Could you check a few things on this model? Use its own coordinates, in mm. A direction names the side the tool comes from. Coordinates: 2 decimals unless noted, no trailing zeros. Order: outer loops, then holes, each group sorted by start corner. A loop starts at its lowest first (then second) coordinate and runs counter-clockwise, first axis right, second up. Notation, with made-up numbers: M 64,43.5 L 94,43.5 A29 cw 94,74.5 Z; hole C -34,36.5 d10. An arc over 180 degrees is marked long. Put each result on its own line as item: value. Start each with the question number.
Autodesk Fusion 360 part; units mm, degrees
sketch "草图1" plane through (0, 0, 0) normal (0, 1, 0) x (1, 0, 0)
  circle A0 centre (0, 0) radius 12
  line L0 (-8.5, -18) -> (8.5, -18)
  line L1 (8.5, -18) -> (15, -4.0607)
  line L2 (-8.5, -18) -> (-15, -4.0607)
  line L3 (0, -38) -> (0, 21) construction
  line L4 (-34, 0) -> (39, 0) construction
  line L5 (-15, 0) -> (-15, -4.0607)
  line L6 (15, 0) -> (15, -4.0607)
  arc A1 (15, 0) -> (-15, 0) centre (0, 0) ccw
  dimension "d1" = 30
  dimension "d2" = 24
  dimension "d3" = 18
  dimension "d4" = 65
  dimension "d5" = 17
extrude "拉伸1" add sketch "草图1" along normal mid plane 30 makes body 1
sketch "草图2" plane through (0, 0, 18) normal (0, 0, 1) x (-1, 0, 0)
  line L0 (-8.5, 15) -> (-8.5, -15)
  line L1 (-8.5, -15) -> (8.5, -15)
  line L2 (8.5, -15) -> (8.5, 15)
  line L3 (8.5, 15) -> (-8.5, 15)
  line L4 (-8.5, 7.5) -> (8.5, 7.5)
  line L5 (8.5, 7.5) -> (8.5, -7.5)
  line L6 (8.5, -7.5) -> (-8.5, -7.5)
  line L7 (-8.5, -7.5) -> (-8.5, 7.5)
  line L8 (-8.5, 7.5) -> (8.5, -7.5) construction
  line L9 (8.5, 7.5) -> (-8.5, -7.5) construction
  dimension "d8" = 15
sketch "草图3" plane through (-15, 0, 0) normal (-1, 0, 0) x (0, -1, 0)
  line L0 (15, 4.0607) -> (-15, 4.0607)
  line L1 (-15, 4.0607) -> (-15, 0)
  line L2 (-15, 0) -> (15, 0)
  line L3 (15, 0) -> (15, 4.0607)
  line L4 (-5, -15) -> (5, -15)
  line L5 (5, -15) -> (5, -5.1421)
  line L6 (-5, -15) -> (-5, -5.1421)
  line L7 (-15, 18) -> (15, 18)
  line L8 (15, 18) -> (15, -15)
  line L9 (15, -15) -> (-15, -15)
  line L10 (-15, -15) -> (-15, 18)
  arc A0 (-5, -5.1421) -> (-15, 9) centre (-20, -5.1421) ccw
  arc A1 (15, 9) -> (5, -5.1421) centre (20, -5.1421) ccw
  line L11 (0, 21) -> (0, -19) construction
  point P0 (15, 18)
  dimension "d9" = 9
  dimension "d10" = 10
  dimension "d11" = 15
extrude "拉伸2" cut sketch "草图3" against normal blind 48 contours L0 L2 L3 L8 A1 | L0 L8 A1 | L2 L5 L8 L9 A1 | L0 L1 L2 L10 A0 | L0 L10 A0 | L2 L6 L9 L10 A0 bodies 1
sketch "草图4" plane through (-15, 0, 0) normal (-1, 0, 0) x (0, -1, 0)
  arc A0 (-5.9089, 0) -> (-8.1548, 4.0607) centre (-20, -5.1421) ccw
  line L0 (-5.9089, 0) -> (5.9089, 0)
  arc A1 (8.1548, 4.0607) -> (5.9089, 0) centre (20, -5.1421) ccw
  line L1 (8.1548, 4.0607) -> (-8.1548, 4.0607)
  line L2 (-15, 18) -> (15, 18)
  line L3 (15, 18) -> (15, 9)
  line L4 (15, 9) -> (-15, 9)
  line L5 (-15, 9) -> (-15, 18)
  line L6 (0, 23) -> (0, -21) construction
  line L7 (-7.5, 18) -> (-17.1867, -2.7731)
  line L8 (-17.1867, -2.7731) -> (17.1867, -2.7731)
  line L9 (17.1867, -2.7731) -> (7.5, 18)
  line L10 (-7.5, 18) -> (7.5, 18)
  line L11 (-15, 18) -> (17.1867, 18)
  line L12 (17.1867, 18) -> (17.1867, -2.7731)
  line L13 (17.1867, -2.7731) -> (-15, -2.7731)
  line L14 (-15, -2.7731) -> (-15, 18)
  dimension "d14" = 15
  dimension "d15" = 65
  dimension "d16" = 65
extrude "拉伸3" cut sketch "草图4" against normal blind 39 contours L2 L4 L5 L7 L11 L14 | L4 L7 L14 | L2 L3 L4 L9 L11 | L3 L4 L9 L11 L12 bodies 1
sketch "草图5" plane through (0, 0, 18) normal (0, 0, 1) x (-1, 0, 0)
  line L0 (6, -5) -> (-6, -5)
  line L1 (-6, -5) -> (-6, 5)
  line L2 (-6, 5) -> (6, 5)
  line L3 (6, 5) -> (6, -5)
  line L4 (6, -5) -> (-6, 5) construction
  line L5 (-6, -5) -> (6, 5) construction
  dimension "d19" = 10
  dimension "d20" = 12
extrude "拉伸4" cut sketch "草图5" against normal blind 5 bodies 1
sketch "草图6" plane through (6, 0, 0) normal (-1, 0, 0) x (0, -1, 0)
  line L0 (5, 18) -> (-5, 18)
  line L1 (-5, 18) -> (-5, 13)
  line L2 (-5, 13) -> (5, 13)
  line L3 (5, 13) -> (5, 18)
  line L4 (-5, 18) -> (-5, 13)
  line L5 (5, 13) -> (5, 18)
  line L6 (-5, 18) -> (-3.6603, 13)
  line L7 (5, 18) -> (3.6603, 13)
  line L8 (5, 13) -> (3.6603, 13)
  line L9 (-3.6603, 13) -> (-5, 13)
  line L10 (0, 22) -> (0, 5.5125) construction
  dimension "d23" = 30
extrude "拉伸5" add sketch "草图6" along normal blind 12 separate body contours L2 L3 L5 L7 L8 | L1 L2 L4 L6 L9 makes body 2 at (2, 4.5534, 16.3333) makes body 3 at (-2, -4.1068, 14.6667)
sketch "草图7" plane through (0, -5, 0) normal (0, 1, 0) x (-1, 0, 0)
  line L0 (6, 18) -> (-6, 18)
  line L1 (-6, 18) -> (-6, 13)
  line L2 (-6, 13) -> (6, 13)
  line L3 (6, 13) -> (6, 18)
  line L4 (-6, 18) -> (-6, 13)
  line L5 (0, 24) -> (0, 4) construction
  line L6 (6, 18) -> (6, 13)
  line L7 (-6, 13) -> (6, 13)
  line L8 (6, 18) -> (4.6603, 13)
  line L9 (-6, 18) -> (-4.6603, 13)
  dimension "d26" = 30
extrude "拉伸6" add sketch "草图7" along normal blind 10 separate body contours L2 L3 L6 L7 L8 | L1 L2 L4 L7 L9 makes body 4 at (5.5534, -1.6667, 16.3333) makes body 5 at (-5.5534, -1.6667, 16.3333)
combine "合并1" operation add target body 1 tool bodies 2 3 5 4
Item 1: If we section it at D-D on z = 14: Write out the boundary of the cut face in (x, y), then the cut area to 3 significant figures.
Item 2: If we section it at B-B on x = -7: Write out the boundary of the cut face in (y, z), then the cut area to 3 significant figures.
Item 3: If we mould it in two halves opening along Y, with no side actions, what happens to faces 1 (the flat face through (0.08, -4.34, 15.54)), 2 (the flat face through (-11.705, -0.172, 11.128)), 3 (the flat face through (-0.19, -9.4, 13.93))? For each: released by +Y, released by -Y, zero draft, split by the parting line, or undercut.
Item 4: If we section it at C-C on y = 10: Write out the boundary of the cut face in (x, z), then the cut area to 3 significant figures.
Item 5: I need wall thicknesses on probe 1 along X at (y, z) = (1.5, 0); probe 2 along Z at (x, y) = (0, 5.25); probe 3 along Z at (x, y) = (1.5, 0.5). Which ranges of each line are inside material? Lowest first, please.
Item 6: For pin 1 Ø5 at (x, z) = (-4, -9) entering from -Y; pin 2 Ø8 at (x, y) = (-8, -8.5) entering from -Z; pin 3 Ø11 at (x, z) = (2.5, -9) entering from +Y; pin 4 Ø5 at (y, z) = (-9, -9.5) entering from -X, each with a flat end and sliding along its axis, tell me the tip position at first contact or that it passes through.
Item 7: For faces 4 (the flat face through (-0.1, 5, -12.3)), 5 (the flat face through (-0.1, -5, -12.3)), 6 (the flat face through (5.34, -0.07, 15.54)), 7 (the flat face through (15, 0, 2)), which set-ups out of +Z, -Z, +X, -X, +Y, -Y let a thin tool reach every point of the face, with its end or its side?
Item 8: If we section it at A-A on z = -9: Write out the boundary of the cut face in (x, y).
Geometry check:
1. outline: M -10.37,-9.37 L 10.37,-9.37 L 10.37,9.37 L -10.37,9.37 Z; hole M -4.93,-3.93 L 4.93,-3.93 L 4.93,3.93 L -4.93,3.93 Z
1. area: 311 mm²
2. outline: M -11.35,9.75 L 11.35,9.75 L 7.5,18 L -7.5,18 Z; M -5,-13.27 L 5,-13.27 L 5,-9.75 L -5,-9.75 Z
2. area: 191 mm²
3. face 1: undercut
3. face 2: zero draft
3. face 3: released by -Y
4. outline: M -14.08,6.04 L -10.37,6.04 A12 cw 10.37,6.04 L 14.08,6.04 L 11,12.64 L -11,12.64 Z
4. area: 77.9 mm²
5. probe 1: x = -15 to -12, 12 to 15
5. probe 2: z = 12 to 18
5. probe 3: z = -14.92 to -11.91, 11.91 to 13
6. pin 1: stops at y = -5
6. pin 2: stops at z = -13.72
6. pin 3: stops at y = 5
6. pin 4: passes through
7. face 4: -Z, +X, -X, +Y
7. face 5: -Z, +X, -X, -Y
7. face 6: +Z
7. face 7: +Z, -Z, +X, +Y, -Y
8. outline: M -12,-5 L -7.94,-5 L -7.94,5 L -12,5 Z; M 7.94,-5 L 12,-5 L 12,5 L 7.94,5 Z
